Autodesk Inventor part; units mm, degrees
ref_plane "YZ Plane" through (0, 0, 0) normal (1, 0, 0) x (0, 1, 0)
ref_plane "XZ Plane" through (0, 0, 0) normal (0, 1, 0) x (-1, 0, 0)
ref_plane "XY Plane" through (0, 0, 0) normal (0, 0, 1) x (1, 0, 0)
sketch "スケッチ1" plane through (0, 0, 0) normal (0, 0, 1) x (1, 0, 0)
  circle A0 centre (0, 0) radius 2
  dimension "d0" = 4
extrude "押し出し1" add sketch "スケッチ1" along normal blind 6
sketch "スケッチ2" plane through (0, 0, 6) normal (0, 0, 1) x (1, 0, 0)
  circle A0 centre (0, 0) radius 2
  circle A1 centre (0, 0) radius 4
  dimension "d3" = 8
extrude "押し出し2" add sketch "スケッチ2" along normal blind 3 contours A0 | A1
fillet "フィレット1" radius 3 1 edges at (-4, 0, 9)
thread "ねじ1"
sketch "スケッチ3" plane through (0, 0, 0) normal (0, 0, -1) x (-1, 0, 0)
  circle A0 centre (0, 0) radius 2
extrude "押し出し3" add sketch "スケッチ3" along normal blind 9
sketch "スケッチ4" plane through (0, 0, 9) normal (0, 0, 1) x (1, 0, 0)
  line L0 (-1.5, 0.866) -> (0, 1.7321)
  line L1 (0, 1.7321) -> (1.5, 0.866)
  line L2 (1.5, 0.866) -> (1.5, -0.866)
  line L3 (1.5, -0.866) -> (0, -1.7321)
  line L4 (0, -1.7321) -> (-1.5, -0.866)
  line L5 (-1.5, -0.866) -> (-1.5, 0.866)
  point P0 (0, 0)
  point P1 (0, 0)
  point P2 (-1.5, 0)
  dimension "d11" = 3
extrude "押し出し4" cut sketch "スケッチ4" against normal blind 2
properties part number "SB　M4 15mm なべネジ (1)" material "Stainless Steel, 440C"
Verification items for the finished model (mm, model axes). A direction names the side the tool comes from. Round coordinates to 2 decimals unless told otherwise and drop trailing zeros. Write each loop counter-clockwise with the first axis right and the second up, starting at its lowest first coordinate (ties: lowest second). Pieces come first, ordered by that corner, then holes. Notation, with made-up numbers: (-35.75, 43) -> (-9.75, 43) arc R18 cw to (-9.75, 49) -> close; hole circle Ø3 at (-4, 7). An arc over 180 degrees is marked (long way). Write each question's results on one line, items separated by ' | '. Start each with the question number.
1. Draft check along Y on faces 3 (the flat face through (0.761, -1.293, 7.993)), 4 (the flat face through (0, 0, -9)). Enter one of: +Y half, -Y half, draft (parallel to the pull), parting line (faces both ways), or undercut.
2. Material ranges on probe 1 along X at (y, z) = (1, 1); probe 2 along Z at (x, y) = (-0.5, -1.25); probe 3 along Y at (x, z) = (0.25, 8), recorded low to high. Write a range as from..to.
3. Depth check by flat-ended pin: P1, Ø2, axis at x = -2, y = -2.5, coming from the -Z side; P2, Ø3, axis at x = -2.5, y = 0, coming from the +Z side; P3, Ø1.9, axis at y = 0, z = 8, coming from the +X side; P4, Ø1.9, axis at y = -0.5, z = 8.5, coming from the -X side. Enter the tip coordinate at first touch or a pass-through.
4. Set-up check for faces 1 (the flat face through (-2, -1, 6)), 2 (the flat face through (0, 0, 7)): record each of +Z, -Z, +X, -X, +Y, -Y from which the full face is reachable in a straight line by a thin tool's end or side.
5. Cross-section at A-A (z = -7.75). Enter the section's corners in (x, y).
Solutions:
1) face 3: undercut | face 4: draft
2) probe 1: x = -1.73..1.73 | probe 2: z = -9..7 | probe 3: y = -3.23..-1.59, 1.59..3.23
3) P1: stops at z = 6 | P2: stops at z = 8.96 | P3: stops at x = 3.81 | P4: stops at x = -3.54
4) face 1: -Z | face 2: +Z
5) outline: circle Ø4 at (0, 0)
